Design review of the part built by this model. Coordinates are the model's own, in mm. A direction names the side the tool comes from. Coordinates: 2 decimals unless noted, no trailing zeros. Loops run counter-clockwise (first coordinate to the right, second up) from the corner with the lowest first, then second, coordinate; pieces in that order, holes last.
Q1. Add section B-B on x = 28. Give the boundary of the cut face in (y, z).
Q2. Add section D-D on x = 22.5. Give the boundary of the cut face in (y, z).
Q3. Wall thickness on probe 1 along X at (y, z) = (40, -2.5); probe 2 along X at (y, z) = (1, -39): over which ranges is each line inside the solid? List them lowest first.
Q4. Machinability: for faces 4 (the face through (18, 3, -25)), 5 (the face through (1, 41.1, -14)), 6 (the face through (52, 1, -25)), which of the approach directions +Z, -Z, +X, -X, +Y, -Y give a long, thin tool a straight path to every point of the face, cutting with its end or side? Answer none if there is none.
Q5. Draft analysis for pull direction Y (two halves, no side actions). For faces 1 (the face through (50.797, 1.521, -1.141)), 2 (the face through (21, 0, -31)), 3 (the face through (1, 36.9, -36)), state which applies: released by +Y, released by -Y, zero draft, split by the parting line, or undercut.
Q6. Add section C-C on z = -14.5. Give the boundary of the cut face in (x, y), and give its area (3 significant figures).
Q7. Add section A-A on y = 11. Give the boundary of the cut face in (x, z), and give its area (3 significant figures).
Q8. For P1, Ø3, axis at y = 35, z = -14.5, coming from the +X side; P2, Ø1.5, axis at x = 1, z = -36.5, coming from the -Y side; P3, Ø3, axis at x = 29, z = -11.5, coming from the +Y side, all flat-tipped, find the tip position at first contact; note any pin that passes through.
```python
from build123d import *

# Parameters (mm, degrees)
SKETCH_1_W          = 52
SKETCH_1_H          = 50
SKETCH_1_R          = 2.1
SKETCH_1_R_2        = 8.75
EXTRUDE_1_DEPTH     = 3
SKETCH_2_W          = 3
SKETCH_2_H          = 50
EXTRUDE_2_DEPTH     = 49
CUT_EXTRUDE_1_DEPTH = 4
FILLET_1_R          = 2
FILLET_2_R          = 2
FILLET_3_R          = 4
FILLET_4_R          = 4
FILLET_5_R          = 4
FILLET_6_R          = 4


with BuildPart() as part:
    # Эскиз1 → Бобышка-Вытянуть1 (new body)
    with BuildSketch(Plane(origin=(0, 0, 0), x_dir=(1, 0, 0), z_dir=(0, 1, 0))):
        with Locations((26, 25)):
            Rectangle(SKETCH_1_W, SKETCH_1_H)
        with Locations(Location((28, 39.5, 0), (0, 0, 270))):
            Circle(SKETCH_1_R, mode=Mode.SUBTRACT)
        with Locations(Location((28, 10.5, 0), (0, 0, 270))):
            Circle(SKETCH_1_R, mode=Mode.SUBTRACT)
        with Locations(Location((28, 25, 0), (0, 0, 270))):
            Circle(SKETCH_1_R_2, mode=Mode.SUBTRACT)
    extrude(amount=EXTRUDE_1_DEPTH)

    # Эскиз2 → Бобышка-Вытянуть2 (add)
    with BuildSketch(Plane(origin=(0, 3, 0), x_dir=(1, 0, 0), z_dir=(0, 1, 0))):
        with Locations((1.5, 25)):
            Rectangle(SKETCH_2_W, SKETCH_2_H)
    extrude(amount=EXTRUDE_2_DEPTH)

    # Эскиз3 → Вырез-Вытянуть1 (cut)
    with BuildSketch(Plane.ZY):
        with BuildLine():
            Line((-39.4, 13.1), (-33.6, 13.1))
            ThreePointArc((-33.6, 13.1), (-31.5, 11), (-33.6, 8.9))
            Line((-33.6, 8.9), (-39.4, 8.9))
            ThreePointArc((-39.4, 8.9), (-41.5, 11), (-39.4, 13.1))
        make_face()
        with BuildLine():
            Line((-16.4, 13.1), (-10.6, 13.1))
            ThreePointArc((-10.6, 13.1), (-8.5, 11), (-10.6, 8.9))
            Line((-10.6, 8.9), (-16.4, 8.9))
            ThreePointArc((-16.4, 8.9), (-18.5, 11), (-16.4, 13.1))
        make_face()
        with BuildLine():
            Line((-16.4, 41.1), (-10.6, 41.1))
            ThreePointArc((-10.6, 41.1), (-8.5, 39), (-10.6, 36.9))
            Line((-10.6, 36.9), (-16.4, 36.9))
            ThreePointArc((-16.4, 36.9), (-18.5, 39), (-16.4, 41.1))
        make_face()
        with BuildLine():
            Line((-39.4, 41.1), (-33.6, 41.1))
            ThreePointArc((-33.6, 41.1), (-31.5, 39), (-33.6, 36.9))
            Line((-33.6, 36.9), (-39.4, 36.9))
            ThreePointArc((-39.4, 36.9), (-41.5, 39), (-39.4, 41.1))
        make_face()
    extrude(amount=-CUT_EXTRUDE_1_DEPTH, mode=Mode.SUBTRACT)

    # Скругление1
    fillet_1_edges = [part.edges().sort_by_distance(p)[0] for p in [
        (3, 3, -25),
    ]]
    fillet(fillet_1_edges, radius=FILLET_1_R)

    # Скругление2
    fillet_2_edges = [part.edges().sort_by_distance(p)[0] for p in [
        (0, 0, -25),
    ]]
    fillet(fillet_2_edges, radius=FILLET_2_R)

    # Скругление3
    fillet_3_edges = [part.edges().sort_by_distance(p)[0] for p in [
        (1.5, 52, 0),
    ]]
    fillet(fillet_3_edges, radius=FILLET_3_R)

    # Скругление4
    fillet_4_edges = [part.edges().sort_by_distance(p)[0] for p in [
        (1.5, 52, -50),
    ]]
    fillet(fillet_4_edges, radius=FILLET_4_R)

    # Скругление5
    fillet_5_edges = [part.edges().sort_by_distance(p)[0] for p in [
        (52, 1.5, 0),
    ]]
    fillet(fillet_5_edges, radius=FILLET_5_R)

    # Скругление6
    fillet_6_edges = [part.edges().sort_by_distance(p)[0] for p in [
        (52, 1.5, -50),
    ]]
    fillet(fillet_6_edges, radius=FILLET_6_R)


solid = part.part
```
Entries:
1. outline: (0, -50) - (3, -50) - (3, -41.6) - (0, -41.6) - close; (0, -37.4) - (3, -37.4) - (3, -33.75) - (0, -33.75) - close; (0, -16.25) - (3, -16.25) - (3, -12.6) - (0, -12.6) - close; (0, -8.4) - (3, -8.4) - (3, 0) - (0, 0) - close
2. outline: (0, -50) - (3, -50) - (3, -31.81) - (0, -31.81) - close; (0, -18.19) - (3, -18.19) - (3, 0) - (0, 0) - close
3. probe 1: x = 0 to 3
3. probe 2: x = 0.27 to 25.96, 30.04 to 52
4. face 4: +Z, -Z, +X, +Y
4. face 5: +X, -X
4. face 6: +Z, -Z, +X, +Y, -Y
5. face 1: zero draft
5. face 2: released by -Y
5. face 3: undercut
6. outline: (0, 2) arc R2 ccw to (2, 0) - (52, 0) - (52, 3) - (5, 3) arc R2 cw to (3, 5) - (3, 8.9) - (0, 8.9) - close; (0, 13.1) - (3, 13.1) - (3, 36.9) - (0, 36.9) - close; (0, 41.1) - (3, 41.1) - (3, 52) - (0, 52) - close
6. area: 278 mm2
7. outline: (0, -50) - (3, -50) - (3, -41.5) - (0, -41.5) - close; (0, -31.5) - (3, -31.5) - (3, -18.5) - (0, -18.5) - close; (0, -8.5) - (3, -8.5) - (3, 0) - (0, 0) - close
7. area: 90.0 mm2
8. P1: stops at x = 3
8. P2: stops at y = 0.02
8. P3: stops at y = 3
